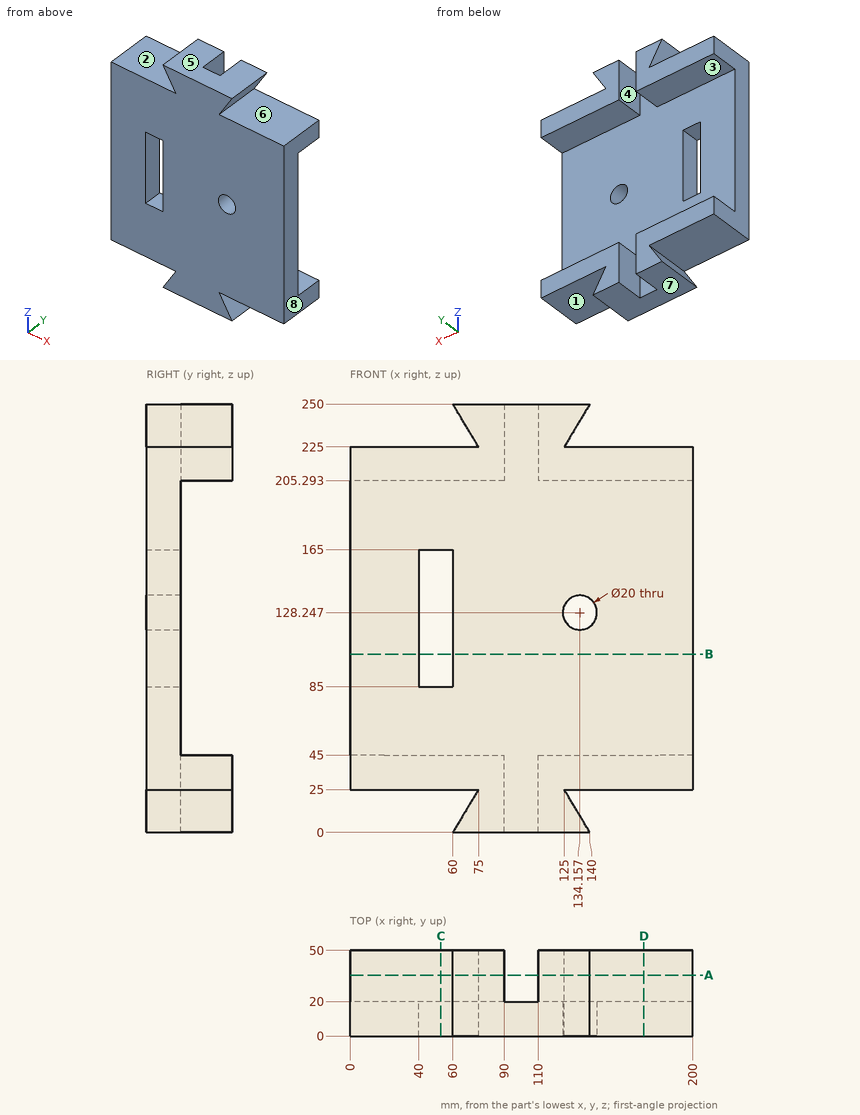
Can you work these out from the drawing? Everything is in mm from the part's minimum corner. A direction names the side the tool comes from. Give positions to 0.01 mm unless a question says otherwise; leave off trailing zeros. Order: outer loops, then holes, each group sorted by start corner. A loop starts at its lowest first (then second) coordinate and runs counter-clockwise, first axis right, second up. Notation, with made-up numbers: M 11,43 L 18,43 A14 cw 18,55 Z; hole C 40,10.25 d11. An arc over 180 degrees is marked long. One line per item, written item: value.
Item 1: For pin 1 (16 mm diameter, centred on x = 134.16, z = 128.25, fed in from +Y); pin 2 (24 mm diameter, centred on x = 28, y = 28.5, fed in from +Z); pin 3 (1.5 mm diameter, centred on x = 165.5, y = 7, fed in from -Z); pin 4 (12 mm diameter, centred on x = 117, z = 143.5, fed in from +Y), each with a flat end and sliding along its axis, tell me the tip position at first contact or that it passes through.
Verdict:
pin 1: through
pin 2: z = 225
pin 3: z = 25
pin 4: y = 20
Item 2: If we section it at A-A on y = 35.5: Write out the boundary of the cut face in (x, z), and give its area (3 significant figures).
Verdict:
outline: M 0,25 L 75,25 L 60,0 L 90,0 L 90,45 L 0,45 Z; M 0,205.29 L 90,205.29 L 90,250 L 60,250 L 75,225 L 0,225 Z; M 110,0 L 140,0 L 125,25 L 200,25 L 200,45 L 110,45 Z; M 110,205.29 L 200,205.29 L 200,225 L 125,225 L 140,250 L 110,250 Z
area: 9,400 mm2
Item 3: If we section it at B-B on z = 104: Write out the boundary of the cut face in (x, y), and give its area (3 significant figures).
Verdict:
outline: M 0,0 L 40,0 L 40,20 L 0,20 Z; M 60,0 L 200,0 L 200,20 L 60,20 Z
area: 3,600 mm2
Item 4: If we section it at D-D on x = 171.5: Write out the boundary of the cut face in (y, z).
Verdict:
outline: M 0,25 L 50,25 L 50,45 L 20,45 L 20,205.29 L 50,205.29 L 50,225 L 0,225 Z
Item 5: Please list where these lines run through material, in increasing order: line 1 (Z direction, x = 148.5, y = 33.5); line 2 (Z direction, x = 113.5, y = 47); line 3 (Z direction, x = 31.5, y = 5.5).
Verdict:
line 1: 25 to 45, 205.29 to 225
line 2: 0 to 45, 205.29 to 250
line 3: 25 to 225
Item 6: If we section it at C-C on x = 53: Write out the boundary of the cut face in (y, z).
Verdict:
outline: M 0,25 L 50,25 L 50,45 L 20,45 L 20,85 L 0,85 Z; M 0,165 L 20,165 L 20,205.29 L 50,205.29 L 50,225 L 0,225 Z
Item 7: For the marked faces 1, 2, 3 and 4, which set-ups out of +Z, -Z, +X, -X, +Y, -Y let a thin tool reach every point of the face, with its end or its side?
Verdict:
face 1: +X, +Y, -Y
face 2: -X, +Y, -Y
face 3: +X, -X, +Y
face 4: +Z, -Z, +Y
Item 8: If we mould it in two halves opening along Z, with no side actions, what happens to the marked faces 5, 6, 7 and 8? For each: pulls with the +Z half, pulls with the -Z half, needs draft (parallel to the pull), parting line crosses it, or undercut.
Verdict:
face 5: pulls with the +Z half
face 6: undercut
face 7: pulls with the -Z half
face 8: needs draft
